Geometry check sheet. Reference: drawing and pictorial views, mm from the part's lowest x, y, z. Give positions to 0.01 mm unless a question says otherwise; leave off trailing zeros. Order: outer loops, then holes, each group sorted by start corner. A loop starts at its lowest first (then second) coordinate and runs counter-clockwise, first axis right, second up. Notation, with made-up numbers: (-36, 66) - (-23, 66) arc R29 ccw to (-23, 91) - close; hole circle Ø1 at (-12, 12). An arc over 180 degrees is marked (long way). Answer in a Markdown table with one row per item.
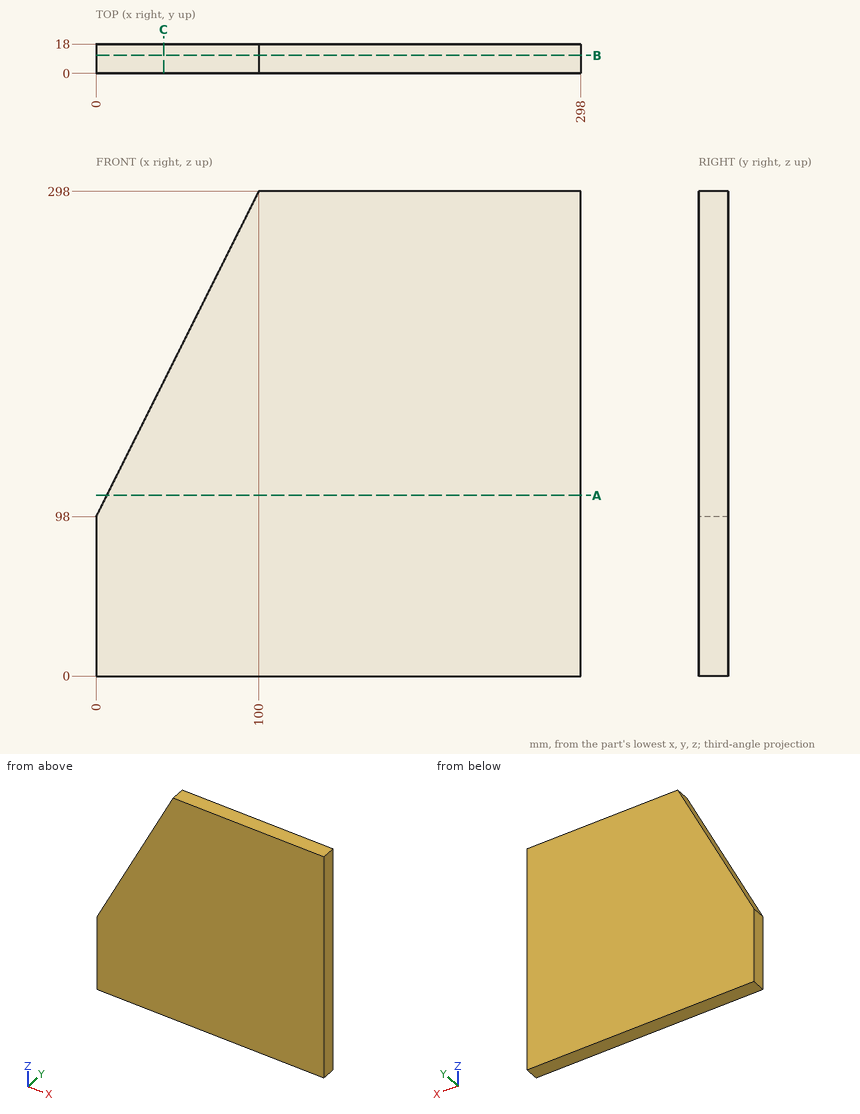
(1) Cross-section at A-A, the plane z = 111. Record the cut outline in (x, y), then the cut area to 3 significant figures.
Geometry says:
| item | result |
|---|---|
| outline | (6.5, 0) - (298, 0) - (298, 18) - (6.5, 18) - close |
| area | 5,250 mm² |
(2) Thickness scan on L1, parallel to X at y = 12.75, z = 182.5; L2, parallel to Z at x = 59, y = 5.75; L3, parallel to X at y = 12, z = 278.5. Record the ranges inside material, lowest first.
Geometry says:
| item | result |
|---|---|
| L1 | 42.25 to 298 |
| L2 | 0 to 216 |
| L3 | 90.25 to 298 |
(3) Cross-section at B-B, the plane y = 11. Record the cut outline in (x, z), then the cut area to 3 significant figures.
Geometry says:
| item | result |
|---|---|
| outline | (0, 0) - (298, 0) - (298, 298) - (100, 298) - (0, 98) - close |
| area | 78,800 mm² |
(4) Gauge pin test, flat ends, axial feed: P1, Ø4, axis at y = 12.5, z = 115, coming from the -X side; P2, Ø5, axis at x = 43, y = 7, coming from the +Z side. Record the tip position at first contact, or that the pin passes through.
Geometry says:
| item | result |
|---|---|
| P1 | x = 7.5 |
| P2 | z = 189 |
(5) Cross-section at C-C, the plane x = 41.5. Record the cut outline in (y, z).
Geometry says:
| item | result |
|---|---|
| outline | (0, 0) - (18, 0) - (18, 181) - (0, 181) - close |
